Build history of the part. All positions in model axes, mm. A direction names the side the tool comes from. Coordinates: 2 decimals unless noted, no trailing zeros. Loops run counter-clockwise (first coordinate to the right, second up) from the corner with the lowest first, then second, coordinate; pieces in that order, holes last. Notation, with made-up numbers: (45, -34.5) - (92, -34.5) arc R14 cw to (92, -9.5) - close; hole circle Ø1 at (-39, 6). An arc over 180 degrees is marked (long way). One line per item, written item: value.
```python
from build123d import *

# Parameters (mm, degrees)
F0_W     = 85
F0_H     = 80
F1_DEPTH = 50
F2_SIZE  = 20
F3_W     = 25
F3_H     = 5
F4_DEPTH = 30
F5_R     = 15
F6_DEPTH = 10
F8_DEPTH = 30


with BuildPart() as f1:
    # F0 (on Top) → F1 (new body)
    with BuildSketch(Plane.XY):
        with Locations((42.5, 40)):
            Rectangle(F0_W, F0_H)
    extrude(amount=F1_DEPTH)

    # F2
    f2_edges = [f1.edges().sort_by_distance(p)[0] for p in [
        (85, 80, 25),
    ]]
    chamfer(f2_edges, length=F2_SIZE)

    # F3 (on face) → F4 (cut)
    with BuildSketch(Plane.XY.offset(50)):
        with Locations((12.5, 77.5)):
            Rectangle(F3_W, F3_H)
    extrude(amount=-F4_DEPTH, mode=Mode.SUBTRACT)

    # F5 (on face) → F6 (join)
    with BuildSketch(Plane.XY.offset(50)):
        with Locations((35, 40)):
            Circle(F5_R)
    extrude(amount=F6_DEPTH)

    # F7 (on face) → F8 (cut)
    with BuildSketch(Plane(origin=(0, 0, 0), x_dir=(1, 0, 0), z_dir=(0, 0, -1))):
        with BuildLine():
            Line((50, 0), (50, -5))
            ThreePointArc((50, -5), (65, -20), (80, -5))
            Line((80, -5), (80, 0))
            Line((80, 0), (50, 0))
        make_face()
    extrude(amount=-F8_DEPTH, mode=Mode.SUBTRACT)


solid = f1.part
```
Item 1: Cut at D-D, the plane z = 38.5. Write the cut outline in (x, y), then the cut area to 4 significant figures.
Check result:
outline: (0, 0) - (85, 0) - (85, 60) - (65, 80) - (25, 80) - (25, 75) - (0, 75) - close
area: 6,475 mm^2
Item 2: Cut at C-C, the plane x = 8. Write the cut outline in (y, z), then the cut area to 3 significant figures.
Check result:
outline: (0, 0) - (80, 0) - (80, 20) - (75, 20) - (75, 50) - (0, 50) - close
area: 3,850 mm^2
Item 3: Pull direction X, two halves, no side cores. Call faces 6 (the face through (80, 3, 15)), 7 (the face through (42, 41, 0)), 8 (the face through (0, 39, 25)): released by +X, released by -X, zero draft, split by the parting line, or undercut.
Check result:
face 6: undercut
face 7: zero draft
face 8: released by -X
Item 4: Cut at B-B, the plane y = 40. Write the cut outline in (x, z), then the cut area to 3 significant figures.
Check result:
outline: (0, 0) - (85, 0) - (85, 50) - (50, 50) - (50, 60) - (20, 60) - (20, 50) - (0, 50) - close
area: 4,550 mm^2
Item 5: Probe probe 1 along Z at (x, y) = (50, 15); probe 2 along Y at (x, z) = (15.5, 46); probe 3 along Z at (x, y) = (62, 7.5). List the from-to ranges inside material, lowest first. Write a range as from..to.
Check result:
probe 1: z = 0..50
probe 2: y = 0..75
probe 3: z = 30..50
Item 6: Drop flat-ended pins along their axis: P1, Ø8, axis at x = 61, z = 7.5, coming from the -Y side; P2, Ø16, axis at x = 61.5, y = 11, coming from the -Z side; P3, Ø1.5, axis at x = 17, z = 28.5, coming from the +Y side. Give the stop position or say it passes through.
Check result:
P1: stops at y = 17.69
P2: stops at z = 30
P3: stops at y = 75
Item 7: Cut at A-A, the plane z = 23.5. Write the cut outline in (x, y).
Check result:
outline: (0, 0) - (50, 0) - (50, 5) arc R15 cw to (80, 5) - (80, 0) - (85, 0) - (85, 60) - (65, 80) - (25, 80) - (25, 75) - (0, 75) - close
Item 8: Tool access for faces 1 (the face through (32, 0, 30)), 2 (the face through (75, 70, 25)), 3 (the face through (23.944, 50.138, 54.93)), 4 (the face through (12, 78, 20)), 5 (the face through (65, 20, 15)): list every direction of +Z, -Z, +X, -X, +Y, -Y with a clear straight run to the whole face (end or side of a thin tool).
Check result:
face 1: +Z, -Z, +X, -X, -Y
face 2: +Z, -Z, +X, +Y
face 3: +Z
face 4: +Z, -X, +Y
face 5: -Z, -Y
